Autodesk Inventor part; units mm, degrees
ref_plane "YZ Plane" through (0, 0, 0) normal (1, 0, 0) x (0, 1, 0)
ref_plane "XZ Plane" through (0, 0, 0) normal (0, 1, 0) x (-1, 0, 0)
ref_plane "XY Plane" through (0, 0, 0) normal (0, 0, 1) x (1, 0, 0)
sketch "Sketch1" plane through (0, 0, 0) normal (0, 0, 1) x (1, 0, 0)
  line L0 (-6.5, 39.5) -> (6.5, 39.5)
  line L1 (6.5, 39.5) -> (6.5, -39.5)
  line L2 (6.5, -39.5) -> (-6.5, -39.5)
  line L3 (-6.5, -39.5) -> (-6.5, 39.5)
  line L4 (-1.5, 39.5) -> (1.5, 39.5)
  line L5 (1.5, 39.5) -> (1.5, 36.5)
  line L6 (1.5, 36.5) -> (-1.5, 36.5)
  line L7 (-1.5, 36.5) -> (-1.5, 39.5)
  line L8 (-6.5, 5) -> (-3.5, 5)
  line L9 (-3.5, 5) -> (-3.5, -5)
  line L10 (-3.5, -5) -> (-6.5, -5)
  line L11 (-6.5, -5) -> (-6.5, 5)
  line L12 (2.5, 39.5) -> (6.5, 39.5)
  line L13 (6.5, 39.5) -> (6.5, -39.5)
  line L14 (6.5, -39.5) -> (2.5, -39.5)
  line L15 (2.5, -39.5) -> (2.5, 39.5) construction
  line L16 (2.5, 15) -> (-6.5, 15)
  line L17 (-6.5, 15) -> (-6.5, 25)
  line L18 (-6.5, 25) -> (2.5, 25)
  line L19 (2.5, 25) -> (2.5, 15)
  line L20 (0, 0) -> (2.358, 0)
  line L21 (2.5, -15) -> (-6.5, -15)
  line L22 (-6.5, -25) -> (2.5, -25)
  line L23 (0, 0) -> (0, 1.2085)
  line L24 (6.5, 5) -> (3.5, 5)
  line L25 (3.5, -5) -> (6.5, -5)
  line L26 (-2.5, 15) -> (6.5, 15)
  line L27 (6.5, 25) -> (-2.5, 25)
  line L28 (-2.5, -15) -> (6.5, -15)
  line L29 (6.5, -25) -> (-2.5, -25)
  line L30 (-3.5, -15) -> (-3.5, -25)
  line L31 (-3.5, 15) -> (-3.5, 25)
  line L32 (3.5, -5) -> (3.5, 5)
  line L33 (3.5, 15) -> (3.5, 25)
  line L34 (3.5, -25) -> (3.5, -15)
  line L35 (-3.5, 25) -> (-3.5, 39.5)
  line L36 (-3.5, 15) -> (-3.5, -39.5)
  line L37 (3.5, -39.5) -> (3.5, 39.5)
  point P0 (0, 39.5)
  point P1 (0, 36.5)
  point P2 (-3.5, 0)
  point P3 (6.5, 0)
  point P4 (-5, 5)
  point P5 (-2, 15)
  point P6 (-2, -15)
  point P7 (5, 5)
  point P8 (2, 15)
  point P9 (2, -15)
  point P10 (-6.5, -25)
  point P11 (2.5, -25)
  point P12 (6.5, -25)
  point P13 (6.5, -25)
  point P14 (6.5, -15)
  point P15 (6.5, -15)
  point P16 (6.5, -5)
  point P17 (6.5, -5)
  point P18 (6.5, 5)
  point P19 (6.5, 5)
  point P20 (6.5, 15)
  point P21 (6.5, 15)
  point P22 (6.5, 25)
  point P23 (6.5, 25)
  point P24 (2.5, 25)
  point P25 (-6.5, 15)
  point P26 (-2, 5)
  point P27 (-6.5, -5)
  point P28 (-2, -5)
  point P29 (2.5, -15)
  point P30 (-6.5, -15)
  point P31 (-3.5, -15)
  point P32 (-3.5, -25)
  point P33 (3.5, -25)
  point P34 (3.5, -15)
  point P35 (3.5, 15)
  point P36 (3.5, 25)
  dimension "d0" = 79
  dimension "d1" = 13
  dimension "d2" = 3
  dimension "d3" = 3
  dimension "d4" = 3
  dimension "d5" = 10
  dimension "d6" = 4
  dimension "d7" = 10
  dimension "d11" = 10
extrude "Extrusion1" add sketch "Sketch1" along normal mid plane 3 contours L0 L7 L6 L5 L37 L27 L18 L35 | L18 L31 L16 L3 | L0 L5 L6 L7 | L18 L19 L16 L31 | L16 L26 L37 L32 L28 L21 L36 L9 | L8 L9 L10 L3 | L27 L33 L26 L19 | L27 L1 L26 L33 | L21 L30 L22 L3 | L21 L28 L34 L29 L22 L30 | L24 L1 L25 L32 | L22 L29 L37 L2 L36 | L28 L1 L29 L34
equation "\"d11\" = d7"
properties part number "Side piece 2x"
The listing builds one solid part. Answer for the finished solid, in the listing's coordinates (mm). A direction names the side the tool comes from. Round coordinates to 2 decimals unless told otherwise and drop trailing zeros. Order: outer loops, then holes, each group sorted by start corner. A loop starts at its lowest first (then second) coordinate and runs counter-clockwise, first axis right, second up. Notation, with made-up numbers: (61, 37.5) -> (78, 37.5) arc R16 cw to (78, 67.5) -> close; hole circle Ø2 at (53.25, 61). An arc over 180 degrees is marked (long way). Answer as CSV lines item,"result".
Q1. A cutting plane is placed at B-B on z = 0.7. Determine the outline of the cut face in (x, y).
Computed values:
outline,"(-6.5, -25) -> (-3.5, -25) -> (-3.5, -39.5) -> (3.5, -39.5) -> (3.5, -25) -> (6.5, -25) -> (6.5, -15) -> (3.5, -15) -> (3.5, -5) -> (6.5, -5) -> (6.5, 5) -> (3.5, 5) -> (3.5, 15) -> (6.5, 15) -> (6.5, 25) -> (3.5, 25) -> (3.5, 39.5) -> (-3.5, 39.5) -> (-3.5, 25) -> (-6.5, 25) -> (-6.5, 15) -> (-3.5, 15) -> (-3.5, 5) -> (-6.5, 5) -> (-6.5, -5) -> (-3.5, -5) -> (-3.5, -15) -> (-6.5, -15) -> close"
Q2. Given pin 1 (0.9 mm diameter, centred on x = -5, z = -0.5, fed in from +Y); pin 2 (0.9 mm diameter, centred on y = -32.5, z = -0.5, fed in from -X); pin 3 (0.9 mm diameter, centred on x = 5.5, z = 0, fed in from -Y), each flat-ended and moving along its own axis, determine where each tip first touches the part or whether it passes through.
Computed values:
pin 1,"stops at y = 25"
pin 2,"stops at x = -3.5"
pin 3,"stops at y = -25"
Q3. For a pull along Y with two mould halves and no side action, classify faces 5 (the flat face through (-3.5, 32, 0)), 6 (the flat face through (-5, 15, 0)), 7 (the flat face through (5, 25, 0)), 8 (the flat face through (5, -25, 0)) as +Y half, -Y half, draft (parallel to the pull), parting line (faces both ways), or undercut.
Computed values:
face 5,"draft"
face 6,"undercut"
face 7,"+Y half"
face 8,"-Y half"
Q4. A cutting plane is placed at C-C on y = -28.5. Determine the outline of the cut face in (x, z).
Computed values:
outline,"(-3.5, -1.5) -> (3.5, -1.5) -> (3.5, 1.5) -> (-3.5, 1.5) -> close"
Q5. A cutting plane is placed at A-A on x = 5.75. Determine the outline of the cut face in (y, z).
Computed values:
outline,"(-25, -1.5) -> (-15, -1.5) -> (-15, 1.5) -> (-25, 1.5) -> close; (-5, -1.5) -> (5, -1.5) -> (5, 1.5) -> (-5, 1.5) -> close; (15, -1.5) -> (25, -1.5) -> (25, 1.5) -> (15, 1.5) -> close"
Q6. Which of the six approach directions +Z, -Z, +X, -X, +Y, -Y give full straight-line access (tool end or side, diameter ignored) to faces 1 (the flat face through (-3.5, -32, 0)), 2 (the flat face through (3.5, -10, 0)), 3 (the flat face through (-6.5, -20, 0)), 4 (the flat face through (-5, 5, 0))?
Computed values:
face 1,"+Z, -Z, -X, -Y"
face 2,"+Z, -Z, +X"
face 3,"+Z, -Z, -X, +Y, -Y"
face 4,"+Z, -Z, -X"
Q7. Consider line 1 (Y direction, x = -4, z = -0.8); line 2 (X direction, y = 10.5, z = 1.1). Determine where each line is inside the solid, lowest interval first. Write a range as from..to.
Computed values:
line 1,"y = -25..-15, -5..5, 15..25"
line 2,"x = -3.5..3.5"
